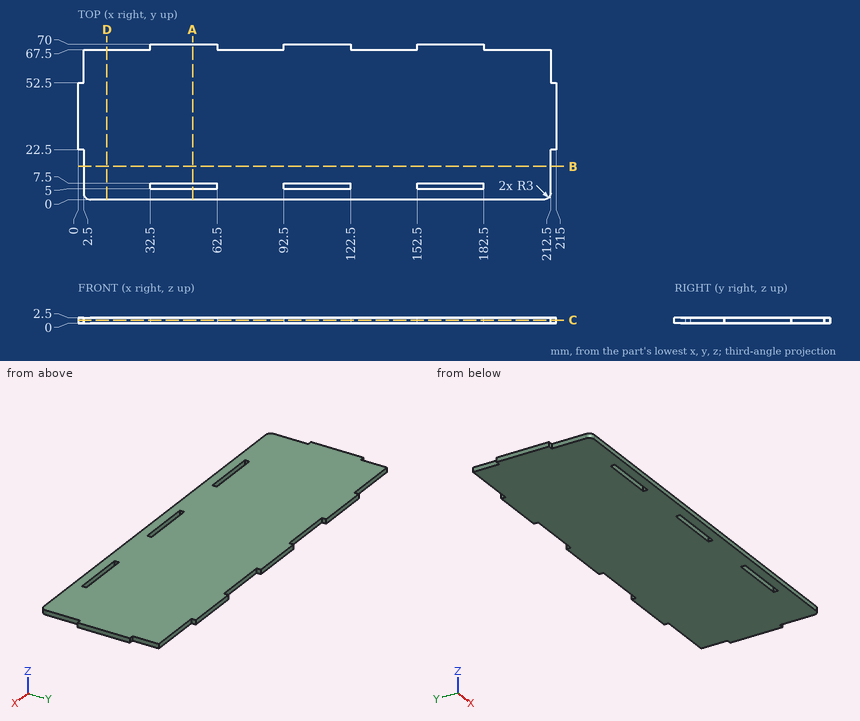
Print and shaded views of the part. All mm, measured from the part's lowest x, y and z. Round coordinates to 2 decimals unless told otherwise and drop trailing zeros. Write each loop counter-clockwise with the first axis right and the second up, starting at its lowest first coordinate (ties: lowest second). Pieces come first, ordered by that corner, then holes. Notation, with made-up numbers: M -29,-14 L -19,-14 A19 cw -19,4 Z; hole C 89,19 d2. An arc over 180 degrees is marked long. Use a Markdown table: item, result. Add a question column.
1. Slice it at A-A on x = 51.5. Give the cut face in (y, z), then the cut area to 3 significant figures.
2. Flat gauge pins, fed straight in: P1, Ø0.8, axis at x = 137.5, z = 1, coming from the +Y side; P2, Ø1.2, axis at y = 56.5, z = 1.5, coming from the -X side; P3, Ø0.8, axis at y = 6, z = 1.5, coming from the +X side. Where does each tip first touch, or does it go through?
3. Slice it at D-D on x = 13. Give the cut face in (y, z), then the cut area to 3 significant figures.
4. Drill centre lines: probe 1 along Y at (x, z) = (158.5, 2.3); probe 2 along Y at (x, z) = (65.5, 1.3); probe 3 along X at (y, z) = (63, 1.95). Where is each one in solid material? Low to high.
5. Slice it at B-B on y = 15. Give the cut face in (x, z).
6. Slice it at C-C on z = 1.45. Give the number of separate pieces and of enclosed holes in the cut face, then the cut area to 3 significant figures.
Reply:
| question | item | result |
|---|---|---|
| 1 | outline | M 0,0 L 5,0 L 5,2.5 L 0,2.5 Z; M 7.5,0 L 70,0 L 70,2.5 L 7.5,2.5 Z |
| 1 | area | 169 mm^2 |
| 2 | P1 | stops at y = 67.5 |
| 2 | P2 | stops at x = 2.5 |
| 2 | P3 | stops at x = 212.5 |
| 3 | outline | M 0,0 L 67.5,0 L 67.5,2.5 L 0,2.5 Z |
| 3 | area | 169 mm^2 |
| 4 | probe 1 | y = 0 to 5, 7.5 to 70 |
| 4 | probe 2 | y = 0 to 67.5 |
| 4 | probe 3 | x = 2.5 to 212.5 |
| 5 | outline | M 2.5,0 L 212.5,0 L 212.5,2.5 L 2.5,2.5 Z |
| 6 | separate pieces | 1 |
| 6 | enclosed holes | 3 |
| 6 | area | 14,300 mm^2 |
